The listing builds one solid part. Answer for the finished solid, in the listing's coordinates (mm). Face numbers are marked on the shaded views. Give positions to 0.01 mm unless a question says otherwise; leave off trailing zeros. Order: outer loops, then holes, each group sorted by start corner. A loop starts at its lowest first (then second) coordinate and runs counter-clockwise, first axis right, second up. Notation, with made-up numbers: (48, 15.25) - (82, 15.25) arc R20 cw to (82, 54.25) - close; hole circle Ø9 at (-12.5, -15.5). An arc over 180 degrees is marked (long way). Answer in a Markdown table with one row per item.
from build123d import *

# Parameters (mm, degrees)
SKETCH_W     = 80
SKETCH_H     = 80
PAD_DEPTH    = 10
SKETCH001_R  = 6
POCKET_DEPTH = 10.001
FILLET_R     = 10


with BuildPart() as part:
    # Sketch → Pad (new body)
    with BuildSketch(Plane.XY):
        Rectangle(SKETCH_W, SKETCH_H)
    extrude(amount=PAD_DEPTH)

    # Sketch001 (on Face6 of Pad) → Pocket (cut, through all)
    with BuildSketch(Plane.XY.offset(10)):
        with Locations((-20, 20)):
            Circle(SKETCH001_R)
        with Locations((20, 20)):
            Circle(SKETCH001_R)
        with Locations((20, -20)):
            Circle(SKETCH001_R)
        with Locations((-20, -20)):
            Circle(SKETCH001_R)
    extrude(amount=-POCKET_DEPTH, mode=Mode.SUBTRACT)

    # Fillet
    fillet_edges = [part.edges().sort_by_distance(p)[0] for p in [
        (-40, -40, 5),
        (40, -40, 5),
        (40, 40, 5),
        (-40, 40, 5),
    ]]
    fillet(fillet_edges, radius=FILLET_R)


solid = part.part
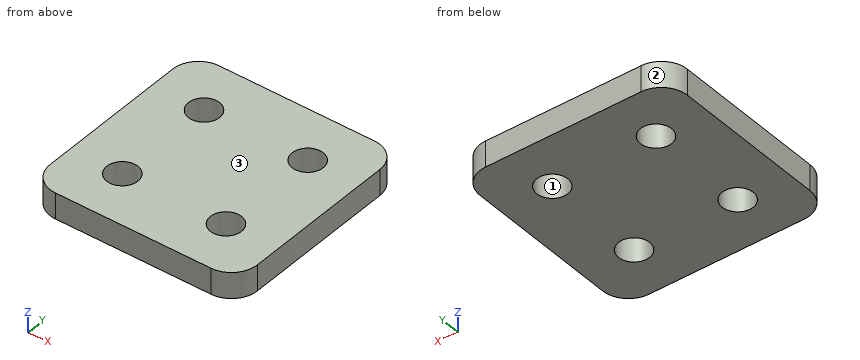
Item 1: Find section A-A on y = -20. Write down the section's boundary in (x, z).
Answer block:
| item | result |
|---|---|
| outline | (-40, 0) - (-26, 0) - (-26, 10) - (-40, 10) - close; (-14, 0) - (14, 0) - (14, 10) - (-14, 10) - close; (26, 0) - (40, 0) - (40, 10) - (26, 10) - close |
Item 2: This flat-tipped pin is pushed along its axis until it touches: P1, Ø11, axis at x = -20, y = -20, coming from the +Z side. Where does it stop, or does it pass through?
Answer block:
| item | result |
|---|---|
| P1 | through |
Item 3: Find section C-C on z = 4.5. Write down the section's boundary in (x, y), then the cut area to 3 significant figures.
Answer block:
| item | result |
|---|---|
| outline | (-40, -30) arc R10 ccw to (-30, -40) - (30, -40) arc R10 ccw to (40, -30) - (40, 30) arc R10 ccw to (30, 40) - (-30, 40) arc R10 ccw to (-40, 30) - close; hole circle Ø12 at (-20, -20); hole circle Ø12 at (-20, 20); hole circle Ø12 at (20, -20); hole circle Ø12 at (20, 20) |
| area | 5,860 mm² |
Item 4: Consider line 1 (Y direction, x = 20, z = 3.5); line 2 (Y direction, x = 17, z = 1.5); line 3 (Y direction, x = -35.5, z = 4.25). Determine where each line is inside the solid, lowest interval first.
Answer block:
| item | result |
|---|---|
| line 1 | -40 to -26, -14 to 14, 26 to 40 |
| line 2 | -40 to -25.2, -14.8 to 14.8, 25.2 to 40 |
| line 3 | -38.35 to 38.35 |
Item 5: Determine the mould class of the marked faces 1, 2 and 3 for opening direction Y: pulls with the +Y half, pulls with the -Y half, needs draft (parallel to the pull), parting line crosses it, or undercut.
Answer block:
| item | result |
|---|---|
| face 1 | undercut |
| face 2 | pulls with the +Y half |
| face 3 | needs draft |
